Here's the drawing with two shaded views (mm, measured from the low corner). I have some questions. A direction names the side the tool comes from. Round coordinates to 2 decimals unless told otherwise and drop trailing zeros. Loops run counter-clockwise (first coordinate to the right, second up) from the corner with the lowest first, then second, coordinate; pieces in that order, holes last.
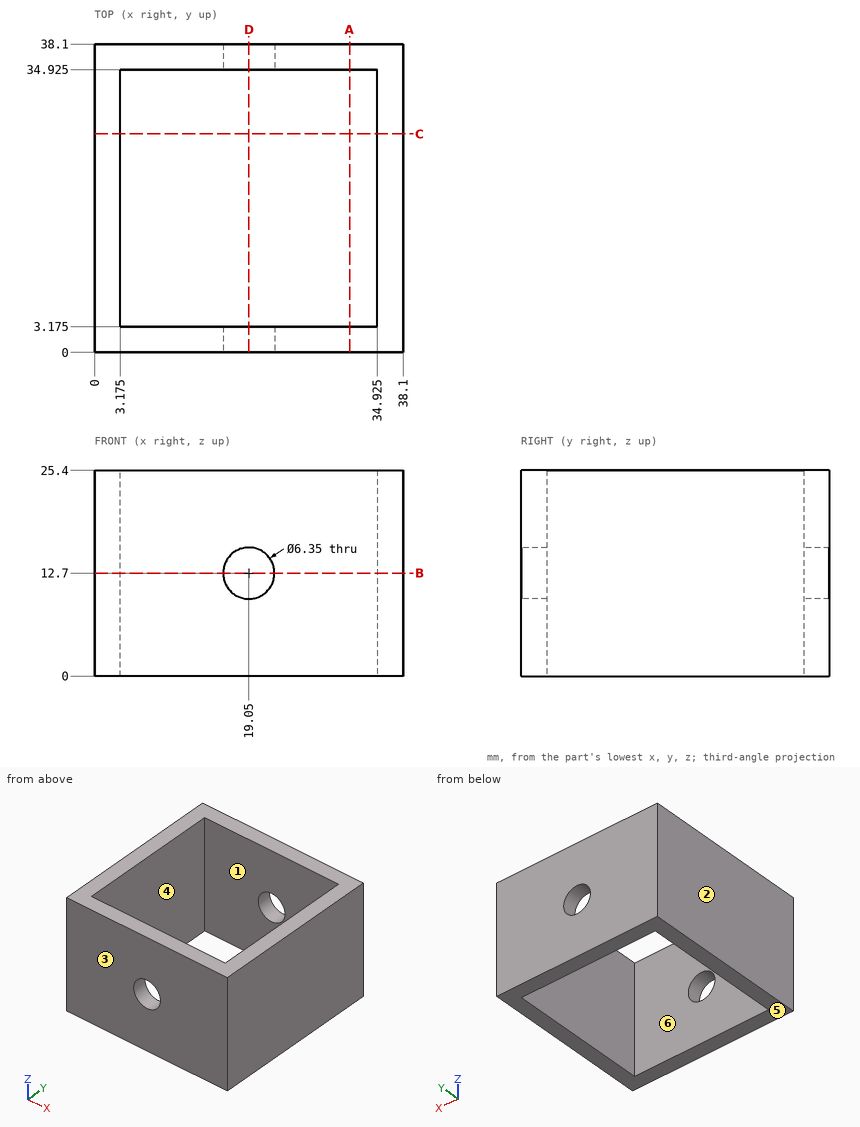
(1) If we section it at D-D, the plane x = 19.05: List the corners of the cut face in (y, z) for me (3 decimals).
Worked answers:
outline: (0, 0) - (3.175, 0) - (3.175, 9.525) - (0, 9.525) - close; (0, 15.875) - (3.175, 15.875) - (3.175, 25.4) - (0, 25.4) - close; (34.925, 0) - (38.1, 0) - (38.1, 9.525) - (34.925, 9.525) - close; (34.925, 15.875) - (38.1, 15.875) - (38.1, 25.4) - (34.925, 25.4) - close
(2) For the marked faces 5 and 6, which set-ups out of +Z, -Z, +X, -X, +Y, -Y let a thin tool reach every point of the face, with its end or its side?
Worked answers:
face 5: -Z, +X, -X, +Y, -Y
face 6: +Z, -Z
(3) If we section it at B-B, the plane z = 12.7: List the corners of the cut face in (x, y) for me (3 decimals), then the cut area to 3 significant figures.
Worked answers:
outline: (0, 0) - (15.875, 0) - (15.875, 3.175) - (3.175, 3.175) - (3.175, 34.925) - (15.875, 34.925) - (15.875, 38.1) - (0, 38.1) - close; (22.225, 0) - (38.1, 0) - (38.1, 38.1) - (22.225, 38.1) - (22.225, 34.925) - (34.925, 34.925) - (34.925, 3.175) - (22.225, 3.175) - close
area: 403 mm2
(4) If we section it at A-A, the plane x = 31.5: List the corners of the cut face in (y, z) for me (3 decimals), then the cut area to 3 significant figures.
Worked answers:
outline: (0, 0) - (3.175, 0) - (3.175, 25.4) - (0, 25.4) - close; (34.925, 0) - (38.1, 0) - (38.1, 25.4) - (34.925, 25.4) - close
area: 161 mm2
(5) If we mould it in two halves opening along X, with no side actions, what happens to the marked faces 1, 2, 3 and 4? For each: released by +X, released by -X, zero draft, split by the parting line, or undercut.
Worked answers:
face 1: undercut
face 2: released by -X
face 3: zero draft
face 4: undercut
(6) If I drill on line 1 (X direction, y = 1.65, z = 12.7) (3 decimals); line 2 (Y direction, x = 12, z = 23) (3 decimals), over which ranges is the centre line in solid material (lowest first)?
Worked answers:
line 1: x = 0 to 15.875, 22.225 to 38.1
line 2: y = 0 to 3.175, 34.925 to 38.1
